Here's the drawing with two shaded views (mm, measured from the low corner). I have some questions. Coordinates: 2 decimals unless noted, no trailing zeros. Write each loop counter-clockwise with the first axis right and the second up, starting at its lowest first coordinate (ties: lowest second). Pieces come first, ordered by that corner, then holes. Notation, with made-up numbers: M 44,13.25 L 89,13.25 A4 ccw 89,17.25 Z; hole C 64,-17.5 d9. An arc over 180 degrees is marked long. Use one line per item in the form item = value. Start each with the question number.
1. I want a section at B-B, the plane x = 80. List the corners of the cut face in (y, z) for me.
2. I want a section at C-C, the plane z = 2.3. List the corners of the cut face in (x, y) for me, plus the area to 3 significant figures.
3. Please list where these lines run through material, in increasing order: line 1 along Y through (x, z) = (21, 1.4); line 2 along X through (y, z) = (38, 5.2); line 3 along X through (y, z) = (35, 1.65). Write a range as [from, to].
4. I want a section at A-A, the plane y = 15. List the corners of the cut face in (x, z) for me, plus the area to 3 significant figures.
5. I want a section at D-D, the plane y = 35. List the corners of the cut face in (x, z) for me, plus the area to 3 significant figures.
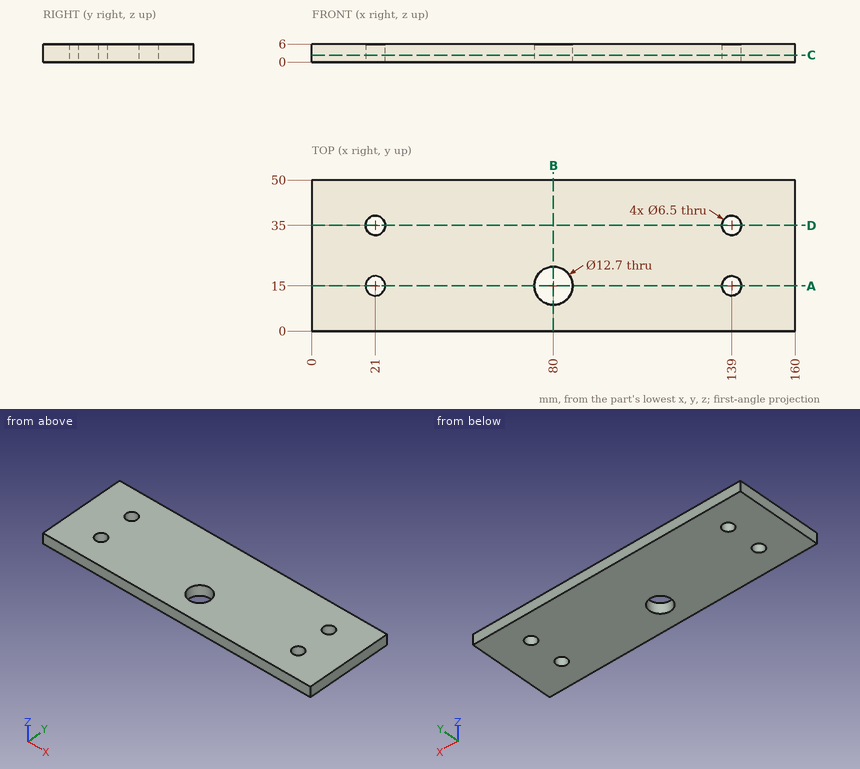
Answer list:
q1.outline = M 0,0 L 8.65,0 L 8.65,6 L 0,6 Z; M 21.35,0 L 50,0 L 50,6 L 21.35,6 Z
q2.outline = M 0,0 L 160,0 L 160,50 L 0,50 Z; hole C 21,15 d6.5; hole C 21,35 d6.5; hole C 80,15 d12.7; hole C 139,15 d6.5; hole C 139,35 d6.5
q2.area = 7,740 mm²
q3.line_1 = [0, 11.75], [18.25, 31.75], [38.25, 50]
q3.line_2 = [0, 19.75], [22.25, 137.75], [140.25, 160]
q3.line_3 = [0, 17.75], [24.25, 135.75], [142.25, 160]
q4.outline = M 0,0 L 17.75,0 L 17.75,6 L 0,6 Z; M 24.25,0 L 73.65,0 L 73.65,6 L 24.25,6 Z; M 86.35,0 L 135.75,0 L 135.75,6 L 86.35,6 Z; M 142.25,0 L 160,0 L 160,6 L 142.25,6 Z
q4.area = 806 mm²
q5.outline = M 0,0 L 17.75,0 L 17.75,6 L 0,6 Z; M 24.25,0 L 135.75,0 L 135.75,6 L 24.25,6 Z; M 142.25,0 L 160,0 L 160,6 L 142.25,6 Z
q5.area = 882 mm²
